Can you work these out from the drawing? Everything is in mm from the part's minimum corner. Round coordinates to 2 decimals unless told otherwise and drop trailing zeros. Order: outer loops, then holes, each group sorted by start corner. A loop starts at its lowest first (then second) coordinate and runs counter-clockwise, first axis right, second up. Notation, with made-up numbers: (77.5, -18.75) - (120.5, -18.75) arc R15 ccw to (120.5, 1.25) - close; hole circle Ø9 at (42, 80.5). An arc over 180 degrees is marked (long way). Write item = value, one per line.
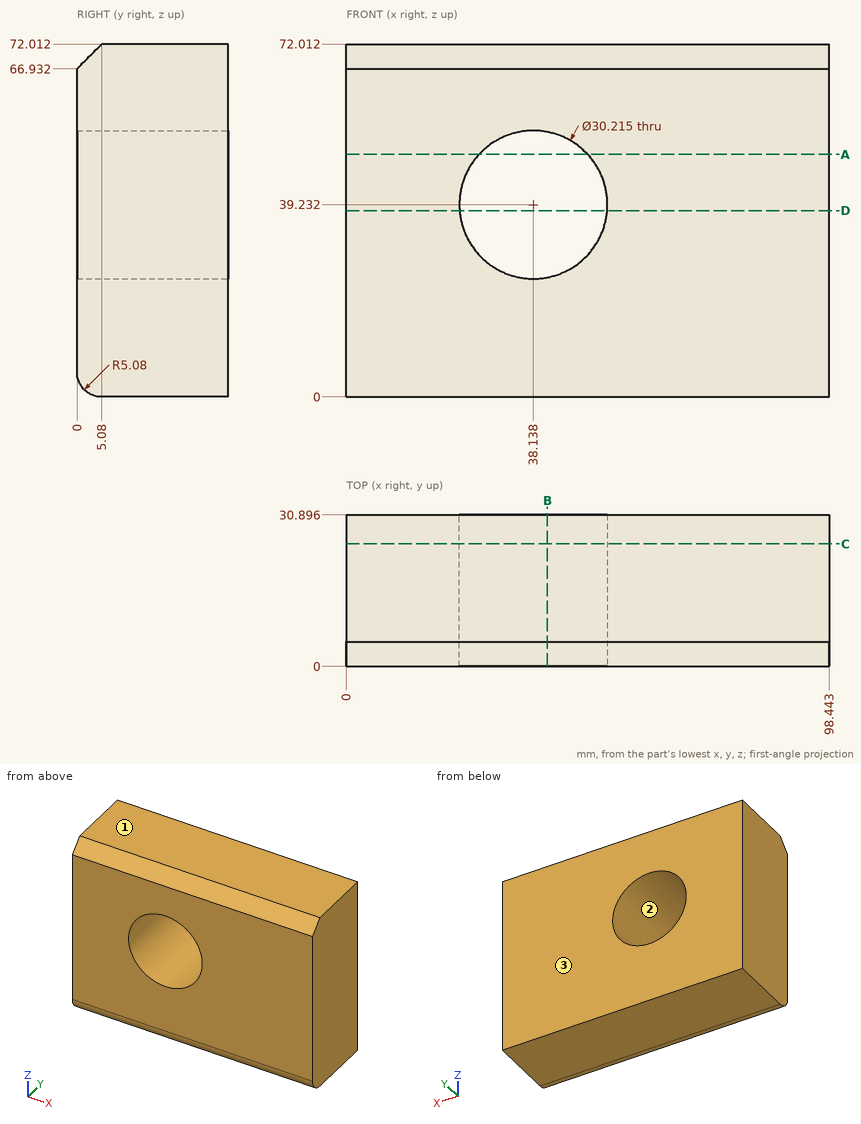
(1) If I drill on line 1 (X direction, y = 22.5, z = 44.5); line 2 (X direction, y = 14.5, z = 49) (1 decimal); line 3 (Z direction, x = 42, y = 29), over which ranges is the centre line in solid material (lowest first)? Write a range as from..to.
Computed:
line_1 = 0..23.98, 52.3..98.44
line_2 = 0..26.6, 49.7..98.4
line_3 = 0..24.63, 53.84..72.01
(2) If we section it at C-C (y = 25): Write out the boundary of the cut face in (x, z) (1 decimal).
Computed:
outline = (0, 0) - (98.4, 0) - (98.4, 72) - (0, 72) - close; hole circle Ø30.2 at (38.1, 39.2)
(3) If we section it at B-B (x = 41): Write out the boundary of the cut face in (y, z) (1 decimal), plus the area to 3 significant figures.
Computed:
outline = (0, 5.1) arc R5.1 ccw to (5.1, 0) - (30.9, 0) - (30.9, 24.4) - (0, 24.4) - close; (0, 54.1) - (30.9, 54.1) - (30.9, 72) - (5.1, 72) - (0, 66.9) - close
area = 1,290 mm^2
(4) If we section it at A-A (z = 49.5): Write out the boundary of the cut face in (x, y) (1 decimal).
Computed:
outline = (0, 0) - (27.1, 0) - (27.1, 30.9) - (0, 30.9) - close; (49.2, 0) - (98.4, 0) - (98.4, 30.9) - (49.2, 30.9) - close
(5) Thinking about a two-plate mould opening in Z: for the marked faces 1, 2 and 3, which applies, +Z half, -Z half, draft (parallel to the pull), parting line (faces both ways), or undercut?
Computed:
face_1 = +Z half
face_2 = undercut
face_3 = draft
(6) If we section it at D-D (z = 38): Write out the boundary of the cut face in (x, y) (1 decimal).
Computed:
outline = (0, 0) - (23.1, 0) - (23.1, 30.9) - (0, 30.9) - close; (53.2, 0) - (98.4, 0) - (98.4, 30.9) - (53.2, 30.9) - close
(7) Will these pins go through, and if not, where does the flat tip stop? P1, Ø3, axis at y = 12, z = 54, coming from the -X side; P2, Ø18, axis at x = 38.14, z = 39.23, coming from the +Y side.
Computed:
P1 = 0
P2 = through
